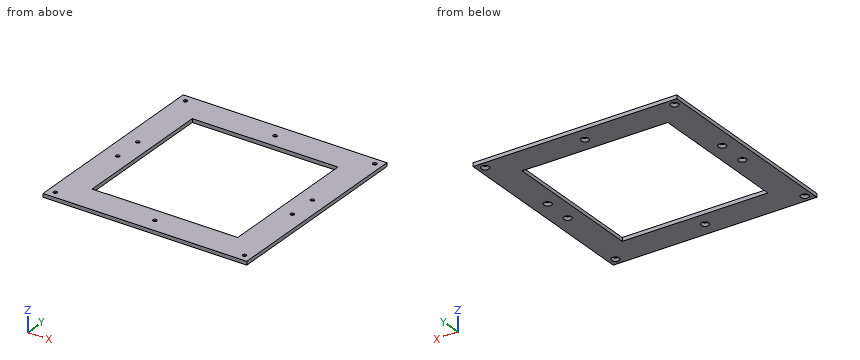
```python
from build123d import *

# Parameters (mm, degrees)
F0_W           = 355.6
F0_H           = 355.6
F0_W_2         = 254
F0_H_2         = 254
F1_DEPTH       = 6.35
F2_D           = 6.7564
F2_DEPTH       = 26.0604
F2_CSINK_D     = 13.4874
F2_CSINK_ANGLE = 82
F2_TIP         = 2.0298273432


# Not quite as in the source:
# - a feature names something its author has since deleted; it is built from what else it names


with BuildPart() as f1:
    # F0 (on Top) → F1 (new body)
    with BuildSketch(Plane.XY):
        with Locations((177.8, 177.8)):
            Rectangle(F0_W, F0_H)
        with Locations((177.8, 177.8)):
            Rectangle(F0_W_2, F0_H_2, mode=Mode.SUBTRACT)
    extrude(amount=F1_DEPTH)

    # F2
    with Locations(Plane(origin=(0, 0, 0), x_dir=(1, 0, 0), z_dir=(0, 0, -1))):
        with Locations((12.7, -342.9), (342.9, -342.9), (342.9, -12.7), (12.7, -12.7), (177.8, -25.4), (177.8, -330.2), (25.4, -152.4), (330.2, -203.2), (330.2, -152.4), (25.4, -203.2)):
            CounterSinkHole(F2_D / 2, F2_CSINK_D / 2, depth=F2_DEPTH, counter_sink_angle=F2_CSINK_ANGLE)
            with Locations((0, 0, -(F2_DEPTH + F2_TIP / 2))):  # 118° drill point
                Cone(0, F2_D / 2, F2_TIP, mode=Mode.SUBTRACT)


solid = f1.part
```
Work out the finished part from the listing and answer in its coordinate system (mm). Coordinates: 2 decimals unless noted, no trailing zeros. Write each loop counter-clockwise with the first axis right and the second up, starting at its lowest first coordinate (ties: lowest second). Pieces come first, ordered by that corner, then holes.
Q1. Find the intervals of material crossed by line 1 (X direction, y = 342.9, z = 5.35); line 2 (X direction, y = 16, z = 2.25); line 3 (Y direction, x = 177.8, z = 5.75), in increasing order.
Q2. A cutting plane is placed at A-A, the plane x = 219.5. Give the vertices of the cut face in (y, z).
Q3. A cutting plane is placed at C-C, the plane z = 2. State how many separate pieces and enclosed holes the cut face has, then the cut area to 3 significant figures.
Q4. Each of these flat-tipped pins is pushed along its axis until it touches: pin 1 Ø3 at (x, z) = (197.5, 4) entering from -Y; pin 2 Ø8 at (x, y) = (177.8, 330.2) entering from -Z; pin 3 Ø11 at (x, y) = (330.2, 152.4) entering from -Z. Where does it stop, or does it pass through?
Findings below:
1. line 1: x = 0 to 9.32, 16.08 to 339.52, 346.28 to 355.6
1. line 2: x = 0 to 9.23, 16.17 to 339.43, 346.37 to 355.6
1. line 3: y = 0 to 22.02, 28.78 to 50.8, 304.8 to 326.82, 333.58 to 355.6
2. outline: (0, 0) - (50.8, 0) - (50.8, 6.35) - (0, 6.35) - close; (304.8, 0) - (355.6, 0) - (355.6, 6.35) - (304.8, 6.35) - close
3. separate pieces: 1
3. enclosed holes: 11
3. area: 61,100 mm2
4. pin 1: stops at y = 0
4. pin 2: stops at z = 3.16
4. pin 3: stops at z = 1.43
